Geometry check sheet. Reference: the model listing, model coordinates, mm. A direction names the side the tool comes from. Give positions to 0.01 mm unless a question says otherwise; leave off trailing zeros. Loops run counter-clockwise (first coordinate to the right, second up) from the corner with the lowest first, then second, coordinate; pieces in that order, holes last. Notation, with made-up numbers: (60.5, 11) -> (85.5, 11) arc R8 cw to (85.5, 21) -> close; hole circle Ø9 at (2, 41.25). An arc over 180 degrees is marked (long way). Answer as a JSON object with one key per item and string values.
from build123d import *

# Parameters (mm, degrees)
SKETCH_1_W             = 55
SKETCH_1_H             = 55
EXTRUDE_1_DEPTH        = 14.5
SKETCH_2_R             = 19.05
CUT_EXTRUDE_1_DEPTH    = 49.512884886
SKETCH_3_W             = 40
SKETCH_3_H             = 35
CUT_EXTRUDE_2_DEPTH    = 32
CHAMFER_1_SIZE         = 3
HOLE_WIZARD_M4_1_D     = 3.3
HOLE_WIZARD_M4_1_DEPTH = 18.5
HOLE_WIZARD_M4_1_TIP   = 0.991420021
HOLE_WIZARD_M4_2_D     = 3.3
HOLE_WIZARD_M4_2_DEPTH = 18.5
HOLE_WIZARD_M4_2_TIP   = 0.991420021
SKETCH_13_W            = 120
SKETCH_13_H            = 55
EXTRUDE_2_DEPTH        = 6
SKETCH_14_W            = 32.5
SKETCH_14_H            = 10
CUT_EXTRUDE_3_DEPTH    = 10
HOLE_START             = -13.1
HOLE_WIZARD_1_DEPTH    = 4.6
HOLE_START_2           = -14.5
HOLE_WIZARD_1_2_DEPTH  = 1.4
FILLET_2_R             = 5


# Read off the part's stored shape, not the designer's step: 打孔尺寸(%根据)内六角圆柱头螺钉的类型1
with BuildPart() as part:
    # 草图1 → 凸台-拉伸1 (new, symmetric)
    with BuildSketch(Plane.XY):
        Rectangle(SKETCH_1_W, SKETCH_1_H)
    extrude(amount=EXTRUDE_1_DEPTH, both=True)

    # 草图2 → 切除-拉伸1 (cut, through all)
    with BuildSketch(Plane(origin=(0, 0, -14.5), x_dir=(-1, 0, 0), z_dir=(0, 0, -1))):
        Circle(SKETCH_2_R)
    extrude(amount=-CUT_EXTRUDE_1_DEPTH, mode=Mode.SUBTRACT)

    # 草图3 → 切除-拉伸2 (cut)
    with BuildSketch(Plane(origin=(-27.5, 0, 0), x_dir=(0, 0, -1), z_dir=(1, 0, 0))):
        Rectangle(SKETCH_3_W, SKETCH_3_H)
    extrude(amount=CUT_EXTRUDE_2_DEPTH, mode=Mode.SUBTRACT)

    # 倒角1
    chamfer_1_edges = [part.edges().sort_by_distance(p)[0] for p in [
        (27.5, -27.5, 0),
        (-27.5, -27.5, 0),
        (-27.5, 27.5, 0),
        (27.5, 27.5, 0),
    ]]
    chamfer(chamfer_1_edges, length=CHAMFER_1_SIZE)

    # M4 螺纹孔1
    with Locations(Plane(origin=(0, 0, -14.5), x_dir=(-1, 0, 0), z_dir=(0, 0, -1))):
        with Locations((-23.5, 23.5), (23.5, 23.5), (23.5, -23.5), (-23.5, -23.5)):
            Hole(HOLE_WIZARD_M4_1_D / 2, depth=HOLE_WIZARD_M4_1_DEPTH)
            with Locations((0, 0, -(HOLE_WIZARD_M4_1_DEPTH + HOLE_WIZARD_M4_1_TIP / 2))):  # 118° drill point
                Cone(0, HOLE_WIZARD_M4_1_D / 2, HOLE_WIZARD_M4_1_TIP, mode=Mode.SUBTRACT)

    # M4 螺纹孔2
    with Locations(Plane.XY.offset(14.5)):
        with Locations((23.5, 23.5), (-23.5, 23.5), (-23.5, -23.5), (23.5, -23.5)):
            Hole(HOLE_WIZARD_M4_2_D / 2, depth=HOLE_WIZARD_M4_2_DEPTH)
            with Locations((0, 0, -(HOLE_WIZARD_M4_2_DEPTH + HOLE_WIZARD_M4_2_TIP / 2))):  # 118° drill point
                Cone(0, HOLE_WIZARD_M4_2_D / 2, HOLE_WIZARD_M4_2_TIP, mode=Mode.SUBTRACT)

    # 草图13 → 凸台-拉伸2 (add)
    with BuildSketch(Plane(origin=(0, 0, -14.5), x_dir=(-1, 0, 0), z_dir=(0, 0, -1))):
        Rectangle(SKETCH_13_W, SKETCH_13_H)
    extrude(amount=-EXTRUDE_2_DEPTH)

    # 草图14 → 切除-拉伸3 (cut)
    with BuildSketch(Plane.XY.offset(-8.5)):
        with Locations((-43.75, -22.5)):
            Rectangle(SKETCH_14_W, SKETCH_14_H)
        with Locations((43.75, -22.5)):
            Rectangle(SKETCH_14_W, SKETCH_14_H)
    extrude(amount=-CUT_EXTRUDE_3_DEPTH, mode=Mode.SUBTRACT)

    # 打孔尺寸(%根据)内六角圆柱头螺钉的类型1 outline → 打孔尺寸(%根据)内六角圆柱头螺钉的类型1 (cut)
    with BuildSketch(Plane.XY.offset(HOLE_START)):
        with BuildLine():
            Line((39.75, -11.5), (50.25, -11.5))
            ThreePointArc((50.25, -11.5), (54.25, -7.5), (50.25, -3.5))
            Line((50.25, -3.5), (39.75, -3.5))
            ThreePointArc((39.75, -3.5), (35.75, -7.5), (39.75, -11.5))
        make_face()
        with BuildLine():
            ThreePointArc((-39.75, -11.5), (-35.75, -7.5), (-39.75, -3.5))
            Line((-39.75, -3.5), (-50.25, -3.5))
            ThreePointArc((-50.25, -3.5), (-54.25, -7.5), (-50.25, -11.5))
            Line((-50.25, -11.5), (-39.75, -11.5))
        make_face()
        with BuildLine():
            Line((39.75, 13.5), (50.25, 13.5))
            ThreePointArc((50.25, 13.5), (54.25, 17.5), (50.25, 21.5))
            Line((50.25, 21.5), (39.75, 21.5))
            ThreePointArc((39.75, 21.5), (35.75, 17.5), (39.75, 13.5))
        make_face()
        with BuildLine():
            ThreePointArc((-39.75, 13.5), (-35.75, 17.5), (-39.75, 21.5))
            Line((-39.75, 21.5), (-50.25, 21.5))
            ThreePointArc((-50.25, 21.5), (-54.25, 17.5), (-50.25, 13.5))
            Line((-50.25, 13.5), (-39.75, 13.5))
        make_face()
    extrude(amount=HOLE_WIZARD_1_DEPTH, mode=Mode.SUBTRACT)

    # Hole Wizard 1 2 outline → Hole Wizard 1 2 (cut)
    with BuildSketch(Plane.XY.offset(HOLE_START_2)):
        with BuildLine():
            Line((39.75, -9.75), (50.25, -9.75))
            ThreePointArc((50.25, -9.75), (52.5, -7.5), (50.25, -5.25))
            Line((50.25, -5.25), (39.75, -5.25))
            ThreePointArc((39.75, -5.25), (37.5, -7.5), (39.75, -9.75))
        make_face()
        with BuildLine():
            ThreePointArc((-39.75, -9.75), (-37.5, -7.5), (-39.75, -5.25))
            Line((-39.75, -5.25), (-50.25, -5.25))
            ThreePointArc((-50.25, -5.25), (-52.5, -7.5), (-50.25, -9.75))
            Line((-50.25, -9.75), (-39.75, -9.75))
        make_face()
        with BuildLine():
            Line((39.75, 15.25), (50.25, 15.25))
            ThreePointArc((50.25, 15.25), (52.5, 17.5), (50.25, 19.75))
            Line((50.25, 19.75), (39.75, 19.75))
            ThreePointArc((39.75, 19.75), (37.5, 17.5), (39.75, 15.25))
        make_face()
        with BuildLine():
            ThreePointArc((-39.75, 15.25), (-37.5, 17.5), (-39.75, 19.75))
            Line((-39.75, 19.75), (-50.25, 19.75))
            ThreePointArc((-50.25, 19.75), (-52.5, 17.5), (-50.25, 15.25))
            Line((-50.25, 15.25), (-39.75, 15.25))
        make_face()
    extrude(amount=HOLE_WIZARD_1_2_DEPTH, mode=Mode.SUBTRACT)

    # 圆角2
    fillet_2_edges = [part.edges().sort_by_distance(p)[0] for p in [
        (60, 27.5, -11.5),
        (-60, 27.5, -11.5),
        (-60, -17.5, -11.5),
        (60, -17.5, -11.5),
    ]]
    fillet(fillet_2_edges, radius=FILLET_2_R)


solid = part.part
1) Section check A-A on x = 0. Record the cut outline in (y, z).
Geometry check:
{"outline": "(-27.5, -14.5) -> (27.5, -14.5) -> (27.5, 14.5) -> (19.05, 14.5) -> (19.05, -8.5) -> (-19.05, -8.5) -> (-19.05, 14.5) -> (-27.5, 14.5) -> close"}
2) Depth check by flat-ended pin: P1, Ø1, axis at x = 23, y = -23.5, coming from the +Z side; P2, Ø1.5, axis at y = -8, z = 7, coming from the +X side; P3, Ø5, axis at x = -42, z = -10, coming from the -Y side. Enter the tip coordinate at first touch or a pass-through.
Geometry check:
{"P1": "stops at z = -8.5", "P2": "stops at x = 27.5", "P3": "stops at y = -17.5"}
3) Draft check along X on faces 1 (the face through (-54.25, 17.59, -10.83)), 2 (the face through (58.57, -16, -11.54)), 3 (the face through (1, 0, -14.5)). Enter one of: pulls with the +X half, pulls with the -X half, needs draft (parallel to the pull), parting line crosses it, or undercut.
Geometry check:
{"face 1": "undercut", "face 2": "pulls with the +X half", "face 3": "needs draft"}
4) Section check B-B on z = 7. Record the cut outline in (x, y).
Geometry check:
{"outline": "(-27.5, -24.5) -> (-24.5, -27.5) -> (24.5, -27.5) -> (27.5, -24.5) -> (27.5, 24.5) -> (24.5, 27.5) -> (-24.5, 27.5) -> (-27.5, 24.5) -> (-27.5, 17.5) -> (-7.53, 17.5) arc R19.05 cw (long way) to (-7.53, -17.5) -> (-27.5, -17.5) -> close; hole circle Ø3.3 at (-23.5, -23.5); hole circle Ø3.3 at (-23.5, 23.5); hole circle Ø3.3 at (23.5, -23.5); hole circle Ø3.3 at (23.5, 23.5)"}
5) Section check C-C on y = 0. Record the cut outline in (x, z).
Geometry check:
{"outline": "(-60, -14.5) -> (60, -14.5) -> (60, -8.5) -> (27.5, -8.5) -> (27.5, 14.5) -> (19.05, 14.5) -> (19.05, -8.5) -> (-60, -8.5) -> close"}
6) Material ranges on line 1 along Y through (x, z) = (23.5, 7.5); line 2 along Y through (x, z) = (-23.5, 7.5), recorded low to high. Write a range as from..to.
Geometry check:
{"line 1": "y = -27.5..-25.15, -21.85..21.85, 25.15..27.5", "line 2": "y = -27.5..-25.15, -21.85..-17.5, 17.5..21.85, 25.15..27.5"}
7) Tool access check on faces 4 (the face through (-23, -23, -8.5)), 5 (the face through (6, 19, 14.5)), 6 (the face through (52.5, 17.5, -13.8)). Record the directions out of +Z, -Z, +X, -X, +Y, -Y that give a thin tool (end or side, any length) a straight path to the whole face; none if there is none.
Geometry check:
{"face 4": "+Z", "face 5": "+Z, +X, -X, +Y, -Y", "face 6": "+Z, -Z"}
8) Section check D-D on x = -34. Record the cut outline in (y, z), plus the area to 3 significant figures.
Geometry check:
{"outline": "(-17.5, -14.5) -> (27.5, -14.5) -> (27.5, -8.5) -> (-17.5, -8.5) -> close", "area": "270 mm2"}
